Geometry: final body of the model. Coordinates: model frame, mm. Face numbers are marked on the shaded views. A direction names the side the tool comes from. Give positions to 0.01 mm unless a question says otherwise; leave off trailing zeros. Loops run counter-clockwise (first coordinate to the right, second up) from the corner with the lowest first, then second, coordinate; pieces in that order, holes last. Notation, with made-up numbers: (-36.5, -26) - (-30.5, -26) arc R12 cw to (-30.5, -14) - close; hole circle Ø3 at (-17.75, 86.25). An arc over 180 degrees is marked (long way). Answer in a Markdown table with one row per item.
from build123d import *

# Parameters (mm, degrees)
F1_DEPTH = 8
F2_DEPTH = 8
F3_START = 5
F3_DEPTH = 3
F4_R     = 50
F5_DEPTH = 5
F7_DEPTH = 5
F8_SIZE  = 3


with BuildPart() as f1:
    # F0 (on Top) → F1 (new body)
    with BuildSketch(Plane.XY):
        with BuildLine():
            ThreePointArc((19.4384842845, -37.7941176471), (36.2793714257, -22.137235802), (42.5, 0))
            ThreePointArc((42.5, 0), (42.488227143, 1.0002770852), (42.4529150943, 2))
            ThreePointArc((42.4529150943, 2), (41.0599774657, 10.969423436), (37.7941176471, 19.4384842845))
            ThreePointArc((37.7941176471, 19.4384842845), (22.137235802, 36.2793714257), (0, 42.5))
            ThreePointArc((0, 42.5), (-1.0002770852, 42.488227143), (-2, 42.4529150943))
            ThreePointArc((-2, 42.4529150943), (-10.969423436, 41.0599774657), (-19.4384842845, 37.7941176471))
            ThreePointArc((-19.4384842845, 37.7941176471), (-36.2793714257, 22.137235802), (-42.5, 0))
            ThreePointArc((-42.5, 0), (-42.488227143, -1.0002770852), (-42.4529150943, -2))
            ThreePointArc((-42.4529150943, -2), (-41.0599774657, -10.969423436), (-37.7941176471, -19.4384842845))
            ThreePointArc((-37.7941176471, -19.4384842845), (-22.137235802, -36.2793714257), (0, -42.5))
            ThreePointArc((0, -42.5), (1.0002770852, -42.488227143), (2, -42.4529150943))
            ThreePointArc((2, -42.4529150943), (10.969423436, -41.0599774657), (19.4384842845, -37.7941176471))
        make_face()
        with BuildLine():
            ThreePointArc((37.5, 0), (8.8235294118, -36.4471580335), (-33.3477508651, -17.1516037805))
            ThreePointArc((-33.3477508651, -17.1516037805), (-8.8235294118, 36.4471580335), (37.5, 0))
        make_face(mode=Mode.SUBTRACT)
    extrude(amount=F1_DEPTH)

    # F0 (on Top) → F2 (join)
    with BuildSketch(Plane.XY):
        with BuildLine():
            ThreePointArc((-47.5, 0), (-47.486842101, -1.1179567422), (-47.4473756936, -2.2352941176))
            Line((-47.4473756936, -2.2352941176), (-42.4529150943, -2))
            ThreePointArc((-42.4529150943, -2), (-42.488227143, -1.0002770852), (-42.5, 0))
            Line((-42.5, 0), (-47.5, 0))
        make_face()
        with BuildLine():
            Line((0, 42.5), (0, 47.5))
            ThreePointArc((0, 47.5), (-1.1179567422, 47.486842101), (-2.2352941176, 47.4473756936))
            Line((-2.2352941176, 47.4473756936), (-2, 42.4529150943))
            ThreePointArc((-2, 42.4529150943), (-1.0002770852, 42.488227143), (0, 42.5))
        make_face()
        with BuildLine():
            Line((42.5, 0), (47.5, 0))
            ThreePointArc((47.5, 0), (47.486842101, 1.1179567422), (47.4473756936, 2.2352941176))
            Line((47.4473756936, 2.2352941176), (42.4529150943, 2))
            ThreePointArc((42.4529150943, 2), (42.488227143, 1.0002770852), (42.5, 0))
        make_face()
        with BuildLine():
            ThreePointArc((0, -47.5), (1.1179567422, -47.486842101), (2.2352941176, -47.4473756936))
            Line((2.2352941176, -47.4473756936), (2, -42.4529150943))
            ThreePointArc((2, -42.4529150943), (1.0002770852, -42.488227143), (0, -42.5))
            Line((0, -42.5), (0, -47.5))
        make_face()
    extrude(amount=F2_DEPTH)

    # F0 (on Top) → F3 (join)
    with BuildSketch(Plane.XY.offset(F3_START)):
        with BuildLine():
            ThreePointArc((-47.4473756936, -2.2352941176), (-45.8905630499, -12.2599438402), (-42.2404844291, -21.7253647886))
            Line((-42.2404844291, -21.7253647886), (-37.7941176471, -19.4384842845))
            ThreePointArc((-37.7941176471, -19.4384842845), (-41.0599774657, -10.969423436), (-42.4529150943, -2))
            Line((-42.4529150943, -2), (-47.4473756936, -2.2352941176))
        make_face()
        with BuildLine():
            ThreePointArc((2.2352941176, -47.4473756936), (12.2599438402, -45.8905630499), (21.7253647886, -42.2404844291))
            Line((21.7253647886, -42.2404844291), (19.4384842845, -37.7941176471))
            ThreePointArc((19.4384842845, -37.7941176471), (10.969423436, -41.0599774657), (2, -42.4529150943))
            Line((2, -42.4529150943), (2.2352941176, -47.4473756936))
        make_face()
        with BuildLine():
            Line((42.4529150943, 2), (47.4473756936, 2.2352941176))
            ThreePointArc((47.4473756936, 2.2352941176), (45.8905630499, 12.2599438402), (42.2404844291, 21.7253647886))
            Line((42.2404844291, 21.7253647886), (37.7941176471, 19.4384842845))
            ThreePointArc((37.7941176471, 19.4384842845), (41.0599774657, 10.969423436), (42.4529150943, 2))
        make_face()
        with BuildLine():
            Line((-2, 42.4529150943), (-2.2352941176, 47.4473756936))
            ThreePointArc((-2.2352941176, 47.4473756936), (-12.2599438402, 45.8905630499), (-21.7253647886, 42.2404844291))
            Line((-21.7253647886, 42.2404844291), (-19.4384842845, 37.7941176471))
            ThreePointArc((-19.4384842845, 37.7941176471), (-10.969423436, 41.0599774657), (-2, 42.4529150943))
        make_face()
    extrude(amount=F3_DEPTH)

    # F4 (on Top) → F5 (join)
    with BuildSketch(Plane.XY):
        Circle(F4_R)
    extrude(amount=-F5_DEPTH)

    # F6 (on Top) → F7 (cut)
    with BuildSketch(Plane.XY):
        with BuildLine():
            Line((-28.3333333333, 9.8601329718), (-47.2222222222, 16.4335549531))
            ThreePointArc((-47.2222222222, 16.4335549531), (-49.3006648592, 8.3333333333), (-50, 0))
            Line((-50, 0), (-30, 0))
            ThreePointArc((-30, 0), (-29.5803989155, 5), (-28.3333333333, 9.8601329718))
        make_face()
    extrude(amount=-F7_DEPTH, mode=Mode.SUBTRACT)

    # F8
    f8_edges = [f1.edges().sort_by_distance(p)[0] for p in [
        (-37.5, 0, 8),
    ]]
    chamfer(f8_edges, length=F8_SIZE)


solid = f1.part
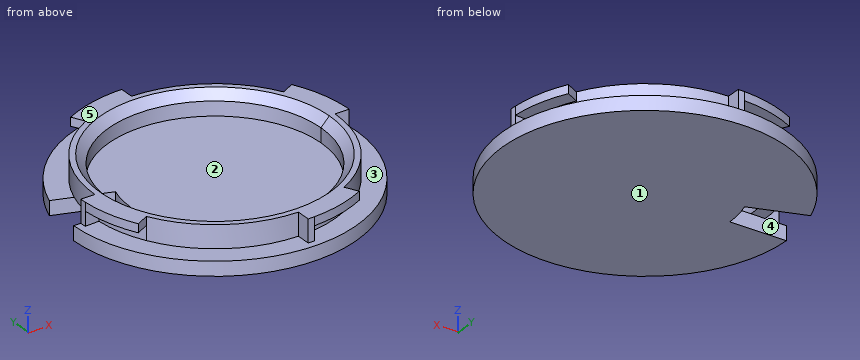
Q1. Cut plane B-B (z = -3.5). Output: boundary loops of the cut face in (x, y), and give its area (3 significant figures).
Check values:
| item | result |
|---|---|
| outline | (-50, 0) arc R50 ccw (long way) to (-47.22, 16.43) - (-28.33, 9.86) arc R30 ccw to (-30, 0) - close |
| area | 7,590 mm² |
Q2. Draft query along X for the marked faces 1 and 2. Return one class per face: pulls with the +X half, pulls with the -X half, needs draft (parallel to the pull), parting line crosses it, or undercut.
Check values:
| item | result |
|---|---|
| face 1 | needs draft |
| face 2 | undercut |
Q3. Reachability of the marked faces 3, 4 and 5 from +Z, -Z, +X, -X, +Y, -Y: full face, straight path, thin tool, end or side. Return the list, or none.
Check values:
| item | result |
|---|---|
| face 3 | none |
| face 4 | -Z, -X |
| face 5 | +Z, +X, -X, +Y, -Y |
Q4. First-contact query: pin 1 (2 mm diameter, centred on x = 17, z = 5.5, fed in from +Y); pin 2 (1 mm diameter, centred on y = 31, z = -2.5, fed in from -X); pin 3 (2.5 mm diameter, centred on y = 45, z = 5.5, fed in from +X). Flat tips, straight axial feed; report the tip coordinate or a pass-through.
Check values:
| item | result |
|---|---|
| pin 1 | y = 39.37 |
| pin 2 | x = -39.62 |
| pin 3 | x = 0 |
Q5. Cut plane A-A (z = 1.5). Output: boundary loops of the cut face in (x, y), and give its area (3 significant figures).
Check values:
| item | result |
|---|---|
| outline | (-47.5, 0) arc R47.5 ccw to (-47.45, -2.24) - (-42.45, -2) arc R42.5 ccw to (0, -42.5) - (0, -47.5) arc R47.5 ccw to (2.24, -47.45) - (2, -42.45) arc R42.5 ccw to (42.5, 0) - (47.5, 0) arc R47.5 ccw to (47.45, 2.24) - (42.45, 2) arc R42.5 ccw to (0, 42.5) - (0, 47.5) arc R47.5 ccw to (-2.24, 47.45) - (-2, 42.45) arc R42.5 ccw to (-42.5, 0) - close; hole circle Ø75 at (0, 0) |
| area | 1,300 mm² |
Q6. Material intervals for line 1 along Z through (x, y) = (43, 18.5); line 2 along Z through (x, y) = (-22.5, 41); line 3 along Y through (x, z) = (0.5, 3.75), sorted ascending.
Check values:
| item | result |
|---|---|
| line 1 | -5 to 0, 5 to 8 |
| line 2 | -5 to 0 |
| line 3 | -47.5 to -37.5, 37.5 to 42.5 |
